Source: CAD feature listing. Evaluate the final solid. Frame: model axes, mm. A direction names the side the tool comes from. Give positions to 0.01 mm unless a question says otherwise; leave off trailing zeros. Order: outer loops, then holes, each group sorted by start corner. A loop starts at its lowest first (then second) coordinate and runs counter-clockwise, first axis right, second up. Notation, with made-up numbers: M -6,-24.5 L 15,-24.5 A29 ccw 15,-2.5 Z; hole C -34,-39 d6. An arc over 180 degrees is marked long. Use CSV: the item, a comma, the result in double quotes. Start each with the question number.
1. Mould query, pull axis Y, two halves, no side actions, for faces 4 (the flat face through (9.2, 14.575, -0.2)), 5 (the cylindrical face through (-2.72, 12.06, -8.63)), 6 (the flat face through (-6, 0, 0)), 7 (the cylindrical face through (-0.246, 4.601, -5.595)). Classes: released by +Y, released by -Y, zero draft, split by the parting line, or undercut.
2. Line query: line 1 along X through (y, z) = (5.25, 0) (3 decimals); line 2 along X through (y, z) = (4, -5); line 3 along Z through (x, y) = (4.5, 7.5). Output: solid intervals per line, ascending. Write a range as [from, to].
3. Pin query (flat end, axial travel): P1, Ø4, axis at x = -2.5, z = 10.5, coming from the +Y side; P2, Ø3.5, axis at x = -0.5, z = -2.5, coming from the -Y side (3 decimals); P3, Ø3, axis at y = 6, z = 1, coming from the -X side. Return the tip coordinate at first contact, or that it passes through.
4. Section query B-B, the plane x = 0. Return the cut outline in (y, z) (3 decimals), plus the area to 3 significant figures.
5. Section query D-D, the plane y = 20.5. Return the cut outline in (x, z), plus the area to 3 significant figures.
6. Section query C-C, the plane y = 13. Return the cut outline in (x, z), plus the area to 3 significant figures.
7. Section query A-A, the plane z = 0. Return the cut outline in (x, y) (3 decimals), plus the area to 3 significant figures.
8. Reachability of faces 1 (the flat face through (0, 22.325, 0)), 2 (the cylindrical face through (7.346, 2.738, 1.631)), 3 (the flat face through (-8, 9.475, -5)) from +Z, -Z, +X, -X, +Y, -Y: full face, straight path, thin tool, end or side. Return the list, or none.
from build123d import *

# Parameters (mm, degrees)
CUT_EXTRUDE_1_DEPTH      = 30.98083763
CUT_EXTRUDE_1_DEPTH_BACK = 9.075
SKETCH_2_R               = 5.6


with BuildPart() as part:
    # Эскиз1 → Повернуть1 (revolve)
    with BuildSketch(Plane.XY, mode=Mode.PRIVATE) as revolve_1_sk:
        Polygon((0, 0), (-7.525, 0), (-7.525, 5.4), (-9.05, 5.4), (-10.525, 9.475), (-9.05, 9.475), (-9.05, 14.575), (-14.15, 14.575), (-14.15, 15.575), (-9.375, 17.325), (-5.525, 22.325), (0, 22.325), align=None)
    revolve(revolve_1_sk.sketch.rotate(Axis((0, 0, 0), (0, 1, 0)), 270), axis=Axis((0, 0, 0), (0, 1, 0)))

    # Эскиз2 → Вырез-Вытянуть1 (cut, two sides: drawn at the far end of the back side and taken through both)
    with BuildSketch(Plane.XZ.offset(-CUT_EXTRUDE_1_DEPTH_BACK)):
        with Locations(Location((0, 0, 0), (0, 0, 90))):
            Circle(SKETCH_2_R)
    extrude(amount=CUT_EXTRUDE_1_DEPTH + CUT_EXTRUDE_1_DEPTH_BACK, mode=Mode.SUBTRACT)


solid = part.part
Result set:
1,face 4,"undercut"
1,face 5,"undercut"
1,face 6,"released by -Y"
1,face 7,"zero draft"
2,line 1,"[-7.525, -5.6], [5.6, 7.525]"
2,line 2,"[-5.62, -2.52], [2.52, 5.62]"
2,line 3,"[-8.72, -3.33], [3.33, 8.72]"
3,P1,"y = 18.08"
3,P2,"y = 9.075"
3,P3,"x = -9.77"
4,outline,"M 0,-7.525 L 5.4,-7.525 L 5.4,-9.05 L 9.475,-10.525 L 9.475,-9.05 L 14.575,-9.05 L 14.575,-14.15 L 15.575,-14.15 L 17.325,-9.375 L 22.325,-5.525 L 22.325,5.525 L 17.325,9.375 L 15.575,14.15 L 14.575,14.15 L 14.575,9.05 L 9.475,9.05 L 9.475,10.525 L 5.4,9.05 L 5.4,7.525 L 0,7.525 L 0,5.6 L 9.075,5.6 L 9.075,-5.6 L 0,-5.6 Z"
4,area,"296 mm2"
5,outline,"C 0,0 d13.86"
5,area,"151 mm2"
6,outline,"C 0,0 d18.1"
6,area,"257 mm2"
7,outline,"M -14.15,14.575 L -9.05,14.575 L -9.05,9.475 L -10.525,9.475 L -9.05,5.4 L -7.525,5.4 L -7.525,0 L -5.6,0 L -5.6,9.075 L 5.6,9.075 L 5.6,0 L 7.525,0 L 7.525,5.4 L 9.05,5.4 L 10.525,9.475 L 9.05,9.475 L 9.05,14.575 L 14.15,14.575 L 14.15,15.575 L 9.375,17.325 L 5.525,22.325 L -5.525,22.325 L -9.375,17.325 L -14.15,15.575 Z"
7,area,"296 mm2"
8,face 1,"+Z, -Z, +X, -X, +Y"
8,face 2,"-Y"
8,face 3,"none"
